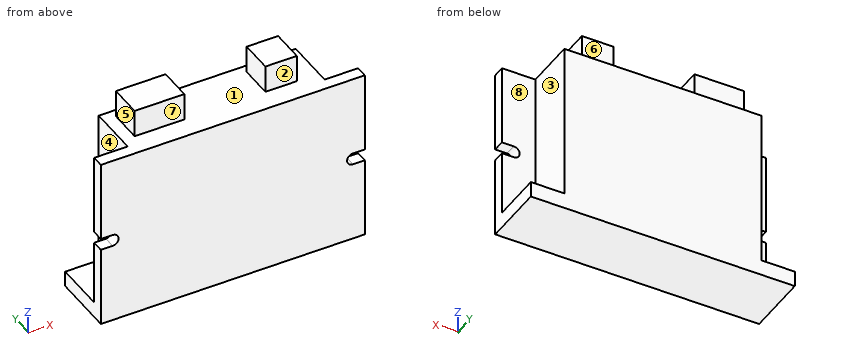
from build123d import *

# Parameters (mm, degrees)
SKETCH2_W               = 85.09
SKETCH2_H               = 55.88
BOSS_EXTRUDE1_DEPTH     = 3.81
SKETCH3_W               = 63.5
SKETCH3_H               = 50.8
BOSS_EXTRUDE2_DEPTH     = 16.51
SKETCH4_W               = 85.09
SKETCH4_H               = 5.08
BOSS_EXTRUDE3_DEPTH     = 16.51
CUT_EXTRUDE1_DEPTH      = 54.509818959
CUT_EXTRUDE1_DEPTH_BACK = 54.509818959
SKETCH6_W               = 16.01364416
SKETCH6_H               = 10.668
SKETCH6_W_2             = 10.127547929
BOSS_EXTRUDE4_DEPTH     = 8.89


with BuildPart() as part:
    # Sketch2 → Boss-Extrude1 (new body)
    with BuildSketch(Plane(origin=(0, 0, 0), x_dir=(1, 0, 0), z_dir=(0, 1, 0))):
        Rectangle(SKETCH2_W, SKETCH2_H)
    extrude(amount=BOSS_EXTRUDE1_DEPTH)

    # Sketch3 → Boss-Extrude2 (add)
    with BuildSketch(Plane(origin=(0, 3.81, 0), x_dir=(1, 0, 0), z_dir=(0, 1, 0))):
        with Locations((0, -2.54)):
            Rectangle(SKETCH3_W, SKETCH3_H)
    extrude(amount=BOSS_EXTRUDE2_DEPTH)

    # Sketch4 → Boss-Extrude3 (add)
    with BuildSketch(Plane(origin=(0, 3.81, 0), x_dir=(1, 0, 0), z_dir=(0, 1, 0))):
        with Locations((0, 25.4)):
            Rectangle(SKETCH4_W, SKETCH4_H)
    extrude(amount=BOSS_EXTRUDE3_DEPTH)

    # Sketch5 → Cut-Extrude1 (cut, two sides: drawn at the far end of the back side and taken through both)
    with BuildSketch(Plane(origin=(0, 3.81, 0), x_dir=(1, 0, 0), z_dir=(0, 1, 0)).offset(-CUT_EXTRUDE1_DEPTH_BACK)):
        with BuildLine():
            Line((38.735, 1.905), (42.545, 1.905))
            Line((42.545, 1.905), (42.545, -1.905))
            Line((42.545, -1.905), (38.735, -1.905))
            ThreePointArc((38.735, -1.905), (36.83, 0), (38.735, 1.905))
        make_face()
        with BuildLine():
            Line((-42.545, 1.905), (-42.545, -1.905))
            Line((-42.545, -1.905), (-38.735, -1.905))
            ThreePointArc((-38.735, -1.905), (-36.83, 0), (-38.735, 1.905))
            Line((-38.735, 1.905), (-42.545, 1.905))
        make_face()
    extrude(amount=CUT_EXTRUDE1_DEPTH + CUT_EXTRUDE1_DEPTH_BACK, mode=Mode.SUBTRACT)

    # Sketch6 → Boss-Extrude4 (add)
    with BuildSketch(Plane.XY.offset(27.94)):
        with Locations((-19.692454306, 12.319)):
            Rectangle(SKETCH6_W, SKETCH6_H)
        with Locations((19.519333829, 12.319)):
            Rectangle(SKETCH6_W_2, SKETCH6_H)
    extrude(amount=BOSS_EXTRUDE4_DEPTH)


solid = part.part
Could you check a few things on this model? Use its own coordinates, in mm. Face numbers are marked on the shaded views. A direction names the side the tool comes from. Coordinates: 2 decimals unless noted, no trailing zeros. Order: outer loops, then holes, each group sorted by start corner. A loop starts at its lowest first (then second) coordinate and runs counter-clockwise, first axis right, second up. Notation, with made-up numbers: (3, -8.75) - (39, -8.75) arc R20 cw to (39, 5.25) - close; hole circle Ø7 at (71.5, 20). An arc over 180 degrees is marked (long way). Answer in a Markdown table with one row per item. Add a question column.
(1) If we section it at C-C, the plane z = 0: Please give me the cut outline in (x, y).
(2) If we section it at D-D, the plane x = 8.5: Please give me the cut outline in (y, z), then the cut area to 3 significant figures.
(3) On a 3-axis mill with a long thin cutter (end or side, diameter ignored), from which of +Z, -Z, +X, -X, +Y, -Y can I reach the whole of each face in a straight line? I mean the marked faces 4, 5, 6, 7 and 8. Say none if no direction works.
(4) If we section it at A-A, the plane x = -26: Please give me the cut outline in (y, z) (3 decimals).
(5) If we mould it in two halves opening along X, with no side actions, what happens to the marked faces 1, 2 and 3? For each: released by +X, released by -X, zero draft, split by the parting line, or undercut.
(6) If we section it at B-B, the plane y = 13.5: Please give me the cut outline in (x, z) (3 decimals).
(7) I need wall thicknesses on L1, parallel to X at y = 9.5, z = 32.5; L2, parallel to X at y = 6.5, z = 27; L3, parallel to Z at x = -7, y = 6.5. Which ranges of each line are inside material? Lowest first, please.
(8) Will these pins go through, and if not, where does the flat tip stop? pin 1 (3 mm diameter, centred on y = 17.5, z = -21, fed in from -X); pin 2 (4.5 mm diameter, centred on y = 11, z = 31, fed in from +X); pin 3 (3 mm diameter, centred on x = 35, y = 15, fed in from +Z).
Results are:
| question | item | result |
|---|---|---|
| 1 | outline | (-36.83, 0) - (36.83, 0) - (36.83, 3.81) - (31.75, 3.81) - (31.75, 20.32) - (-31.75, 20.32) - (-31.75, 3.81) - (-36.83, 3.81) - close |
| 2 | outline | (0, -27.94) - (20.32, -27.94) - (20.32, 27.94) - (0, 27.94) - close |
| 2 | area | 1,140 mm2 |
| 3 | face 4 | +Z, -X, +Y |
| 3 | face 5 | +Z, -X, +Y, -Y |
| 3 | face 6 | +Z, +X, -X, +Y |
| 3 | face 7 | +Z, +X, -X, -Y |
| 3 | face 8 | +Z, +X, +Y |
| 4 | outline | (0, -27.94) - (20.32, -27.94) - (20.32, 27.94) - (17.653, 27.94) - (17.653, 36.83) - (6.985, 36.83) - (6.985, 27.94) - (0, 27.94) - close |
| 5 | face 1 | undercut |
| 5 | face 2 | zero draft |
| 5 | face 3 | released by +X |
| 6 | outline | (-42.545, -27.94) - (42.545, -27.94) - (42.545, -22.86) - (31.75, -22.86) - (31.75, 27.94) - (24.583, 27.94) - (24.583, 36.83) - (14.456, 36.83) - (14.456, 27.94) - (-11.686, 27.94) - (-11.686, 36.83) - (-27.699, 36.83) - (-27.699, 27.94) - (-31.75, 27.94) - (-31.75, -22.86) - (-42.545, -22.86) - close |
| 7 | L1 | x = -27.7 to -11.69, 14.46 to 24.58 |
| 7 | L2 | x = -31.75 to 31.75 |
| 7 | L3 | z = -27.94 to 27.94 |
| 8 | pin 1 | stops at x = -31.75 |
| 8 | pin 2 | stops at x = 24.58 |
| 8 | pin 3 | stops at z = -22.86 |
